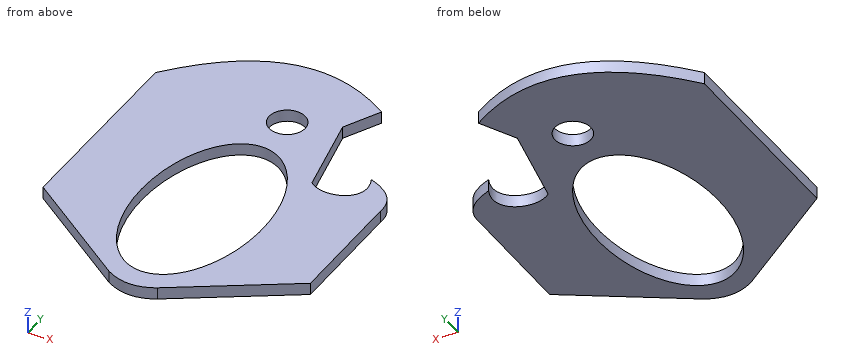
```python
from build123d import *

# Parameters (mm, degrees)
BOSS_EXTRUDE1_DEPTH = 2
SKETCH2_R           = 3
CUT_EXTRUDE1_DEPTH  = 44.941077942
SKETCH3_RX          = 17.5
SKETCH3_RY          = 10
CUT_EXTRUDE2_DEPTH  = 44.941077942


with BuildPart() as part:
    # Sketch1 → Boss-Extrude1 (new body)
    with BuildSketch(Plane.XY):
        with BuildLine():
            Line((10.5, 33.5), (7.5, 27.5))
            Line((7.5, 27.5), (10.5, 13.5))
            add(Edge.make_bspline(
                [(10.5, 13.5), (13.496182411, 11.027569171), (20.037267901, 13.306377108), (17.5, 18.5)],
                knots=[0, 0, 0, 0, 1, 1, 1, 1], degree=3))
            add(Edge.make_bspline(
                [(17.5, 18.5), (22.853553391, 16.681980515), (22.5, 12.5)],
                knots=[0, 0, 0, 1, 1, 1], degree=2))
            Line((22.5, 12.5), (22.62041986, -7.841479807))
            Line((22.62041986, -7.841479807), (4.12041986, -19.841479807))
            add(Edge.make_bspline(
                [(-3.970513587, -19.841479807), (0.071073188, -22.212443979), (4.12041986, -19.841479807)],
                knots=[0, 0, 0, 1, 1, 1], degree=2))
            Line((-3.970513587, -19.841479807), (-22.5, -6.845777179))
            Line((-22.5, -6.845777179), (-22.5, -4.500101611))
            Line((-22.5, -4.500101611), (-22.5, 25.5))
            add(Edge.make_bspline(
                [(-22.5, 25.5), (-6.957614564, 44.682729257), (10.5, 33.5)],
                knots=[0, 0, 0, 1, 1, 1], degree=2))
        make_face()
    extrude(amount=BOSS_EXTRUDE1_DEPTH)

    # Sketch2 → Cut-Extrude1 (cut, through all)
    with BuildSketch(Plane.XY.offset(2)):
        with Locations((0, 24.5)):
            Circle(SKETCH2_R)
    extrude(amount=-CUT_EXTRUDE1_DEPTH, mode=Mode.SUBTRACT)

    # Sketch3 → Cut-Extrude2 (cut, through all)
    with BuildSketch(Plane.XY.offset(2)):
        with Locations(Location((0, 0), (0, 0, -90))):
            Ellipse(SKETCH3_RX, SKETCH3_RY)
    extrude(amount=-CUT_EXTRUDE2_DEPTH, mode=Mode.SUBTRACT)


solid = part.part
```
The listing builds one solid part. Answer for the finished solid, in the listing's coordinates (mm). Round coordinates to 2 decimals unless told otherwise and drop trailing zeros. Loops run counter-clockwise (first coordinate to the right, second up) from the corner with the lowest first, then second, coordinate; pieces in that order, holes last. Notation, with made-up numbers: (-25, 25) - (-8, 25) arc R19 ccw to (-8, 30) - close; hole circle Ø3 at (32, 13). An arc over 180 degrees is marked (long way). Return JSON: item names as keys, results as strings. Group by question number.
1. The part is cut by section A-A on y = 24.5. Determine the outline of the cut face in (x, z), then the cut area to 3 significant figures.
2. Consider probe 1 along X at (y, z) = (16.5, 0.2); probe 2 along Y at (x, z) = (4, 0.8); probe 3 along X at (y, z) = (-5, 1.85). Determine where each line is inside the solid, lowest interval first.
3. The part is cut by section B-B on z = 0.5. State how many separate pieces and enclosed holes the cut face has, then the cut area to 3 significant figures.
Resolved:
{
 "1": {"outline": "(-22.5, 0) - (-3, 0) - (-3, 2) - (-22.5, 2) - close; (3, 0) - (8.14, 0) - (8.14, 2) - (3, 2) - close", "area": "49.3 mm²"},
 "2": {"probe 1": "x = -22.5 to -3.33, 3.33 to 9.86, 18.07 to 21.05", "probe 2": "y = -19.91 to -16.04, 16.04 to 36.63", "probe 3": "x = -22.5 to -9.58, 9.58 to 22.6"},
 "3": {"separate pieces": "1", "enclosed holes": "2", "area": "1,380 mm²"}
}
